Can you work these out from the model? Positions are in its coordinate system, mm. Face numbers are marked on the shaded views. A direction names the side the tool comes from. Coordinates: 2 decimals unless noted, no trailing zeros. Loops run counter-clockwise (first coordinate to the right, second up) from the corner with the lowest first, then second, coordinate; pieces in that order, holes last.
```python
from build123d import *

# Parameters (mm, degrees)
SKETCH_1_R          = 26
EXTRUDE_1_DEPTH     = 3
SKETCH_2_R          = 8.75
EXTRUDE_2_DEPTH     = 25
SKETCH_3_R          = 6.25
CUT_EXTRUDE_1_DEPTH = 28
SKETCH_5_R          = 1.6
CUT_EXTRUDE_3_DEPTH = 3


with BuildPart() as part:
    # 草图1 → 凸台-拉伸1 (new body)
    with BuildSketch(Plane(origin=(0, 0, 0), x_dir=(1, 0, 0), z_dir=(0, 1, 0))):
        with Locations(Location((0, 0, 0), (0, 0, 270))):
            Circle(SKETCH_1_R)
    extrude(amount=EXTRUDE_1_DEPTH)

    # 草图2 → 凸台-拉伸2 (add)
    with BuildSketch(Plane(origin=(0, 3, 0), x_dir=(1, 0, 0), z_dir=(0, 1, 0))):
        with Locations(Location((0, 0, 0), (0, 0, 270))):
            Circle(SKETCH_2_R)
    extrude(amount=EXTRUDE_2_DEPTH)

    # 草图3 → 切除-拉伸1 (cut)
    with BuildSketch(Plane(origin=(0, 28, 0), x_dir=(1, 0, 0), z_dir=(0, 1, 0))):
        with Locations(Location((0, 0, 0), (0, 0, 270))):
            Circle(SKETCH_3_R)
    extrude(amount=-CUT_EXTRUDE_1_DEPTH, mode=Mode.SUBTRACT)

    # 草图5 → 切除-拉伸3 (cut)
    with BuildSketch(Plane.XZ):
        with Locations(Location((0, 20, 0), (0, 0, 270))):
            Circle(SKETCH_5_R)
        with Locations(Location((17.320508076, -10, 0), (0, 0, 270))):
            Circle(SKETCH_5_R)
        with Locations(Location((-17.320508076, -10, 0), (0, 0, 270))):
            Circle(SKETCH_5_R)
    extrude(amount=-CUT_EXTRUDE_3_DEPTH, mode=Mode.SUBTRACT)


solid = part.part
```
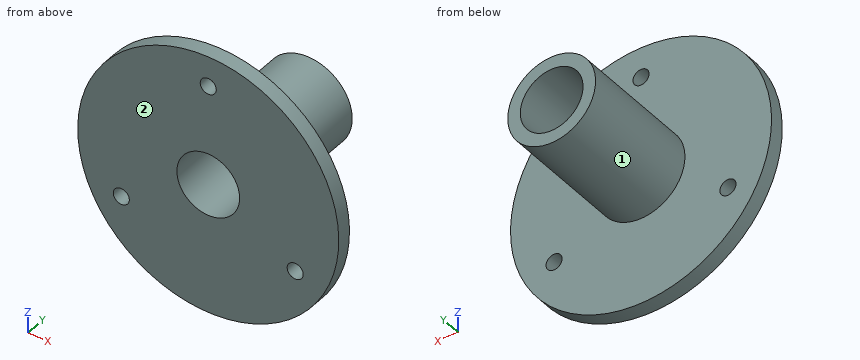
Item 1: Suppose I cut it at C-C, the plane z = -10. Please give me the cut outline in (x, y).
Results are:
outline: (-24, 0) - (-18.92, 0) - (-18.92, 3) - (-24, 3) - close; (-15.72, 0) - (15.72, 0) - (15.72, 3) - (-15.72, 3) - close; (18.92, 0) - (24, 0) - (24, 3) - (18.92, 3) - close
Item 2: Suppose I cut it at B-B, the plane z = 0. Please give me the cut outline in (x, y), plus the area to 4 significant figures.
Results are:
outline: (-26, 0) - (-6.25, 0) - (-6.25, 28) - (-8.75, 28) - (-8.75, 3) - (-26, 3) - close; (6.25, 0) - (26, 0) - (26, 3) - (8.75, 3) - (8.75, 28) - (6.25, 28) - close
area: 243.5 mm2
Item 3: I'm going to push flat-ended pins straight in: P1, Ø6, axis at x = 9, z = 9, coming from the +Y side; P2, Ø1.5, axis at y = 16, z = 7.5, coming from the +X side; P3, Ø5, axis at y = 20.5, z = 7, coming from the -X side. Where does each tip first touch, or does it pass through?
Results are:
P1: stops at y = 3
P2: stops at x = 5.57
P3: stops at x = -7.5
Item 4: On a 3-axis mill with a long thin cutter (end or side, diameter ignored), from which of +Z, -Z, +X, -X, +Y, -Y can I reach the whole of each face in a straight line? I mean the marked faces 1 and 2. Say none if no direction works.
Results are:
face 1: +Y
face 2: +Z, -Z, +X, -X, -Y
Item 5: I need wall thicknesses on line 1 along X through (y, z) = (1.15, -10); line 2 along Y through (x, z) = (-7.5, 12.5); line 3 along X through (y, z) = (7, 0). Which ranges of each line are inside material? Lowest first, please.
Results are:
line 1: x = -24 to -18.92, -15.72 to 15.72, 18.92 to 24
line 2: y = 0 to 3
line 3: x = -8.75 to -6.25, 6.25 to 8.75
Item 6: Suppose I cut it at A-A, the plane x = 0. Please give me the cut outline in (y, z), plus the area to 3 significant figures.
Results are:
outline: (0, -26) - (3, -26) - (3, -8.75) - (28, -8.75) - (28, -6.25) - (0, -6.25) - close; (0, 6.25) - (28, 6.25) - (28, 8.75) - (3, 8.75) - (3, 18.4) - (0, 18.4) - close; (0, 21.6) - (3, 21.6) - (3, 26) - (0, 26) - close
area: 234 mm2
Item 7: Suppose I cut it at D-D, the plane x = 18. Please give me the cut outline in (y, z), plus the area to 3 significant figures.
Results are:
outline: (0, -18.76) - (3, -18.76) - (3, -11.45) - (0, -11.45) - close; (0, -8.55) - (3, -8.55) - (3, 18.76) - (0, 18.76) - close
area: 104 mm2
